Autodesk Inventor part; units mm, degrees
ref_plane "Work Plane1" through (30, 0, 0) normal (0, -0.5, 0.866) x (1, 0, 0)
ref_plane "YZ Plane" through (0, 0, 0) normal (1, 0, 0) x (0, 1, 0)
ref_plane "XZ Plane" through (0, 0, 0) normal (0, 1, 0) x (-1, 0, 0)
sketch "Sketch1" plane through (0, 0, 0) normal (0, 0, 1) x (1, 0, 0)
  line L0 (0.1133, 0) -> (20, 0)
  line L1 (20, 0) -> (20, 3)
  line L2 (20, 3) -> (2, 3)
  line L3 (2, 3) -> (1.3865, 3)
  line L4 (1.3865, 3) -> (0, 3)
  line L5 (0, 3) -> (0, 5.25)
  line L6 (0, 5.25) -> (-3.3, 5.25)
  line L7 (-3.3, 5.25) -> (-3.3, 2.3094)
  line L8 (-3.3, 2.3094) -> (-1.22, 2.3094)
  line L9 (-1.22, 2.3094) -> (0.1133, 0)
  line L10 (-7.96, 0) -> (24.66, 0)
  line L11 (0, -1.05) -> (0, 6.3)
  line L12 (2, 3) -> (0, 3) construction
  dimension "d0" = 18
  dimension "d1" = 0.6135
  dimension "d2" = 3.3
  dimension "d3" = 2.08
  dimension "d4" = 60
  dimension "d5" = 6
  dimension "d6" = 6
  dimension "d7" = 4.6188
  dimension "d8" = 10.5
  dimension "d19" = 20
revolve "Body" add sketch "Sketch1" angle 360 about axis through (0.1133, 0, 0) along (1, 0, 0) contours L9 L11 L4 L3 L2 L1 L0 | L9 L8 L7 L6 L5 L11
sketch "Sketch2" plane through (-3.3, 0, 0) normal (-1, 0, 0) x (0, 0, 1)
  circle A0 centre (0, 0) radius 2.3094
  line L0 (0, -7.35) -> (0, 7.35)
  line L1 (-7.35, 0) -> (7.35, 0)
  line L2 (2.3094, 0) -> (1.1547, -2)
  line L3 (1.1547, -2) -> (-1.1547, -2)
  line L4 (-1.1547, -2) -> (-2.3094, 0)
  line L5 (-2.3094, 0) -> (-1.1547, 2)
  line L6 (-1.1547, 2) -> (1.1547, 2)
  line L7 (1.1547, 2) -> (2.3094, 0)
extrude "Slot" add sketch "Sketch2" against normal up to next contours L7 A0 | A0 L2 | L6 L0 A0 | A0 L0 L3 | L0 L6 A0 | A0 L3 L0 | L4 A0 | A0 L5
fillet "Fillet1" radius 2.5 1 edges at (-3.3, -5.25, 0)
thread "Thread"
chamfer "Chamfer1" distance 0.6135 distance2 0.6135 1 edges at (20, -3, 0) measured on face at (20, 1.0659, 1.0214)
fillet "Fillet2" radius 0.25 1 edges at (0, -3, 0)
ref_plane "Work Plane1" through (30, 0, 0) normal (0, -0.5, 0.866) x (1, 0, 0)
equation "\"d0\" = GEL"
equation "\"d1\" = GAL"
equation "\"d2\" = KOH"
equation "\"d3\" = INTI"
equation "\"d5\" = GD"
equation "\"d6\" = BDM"
equation "\"d7\" = 1.1547 * SW"
equation "\"d8\" = KOD"
equation "\"d19\" = NLG"
equation "\"d16\" = RR"
equation "\"d12\" = GEL"
equation "\"d14\" = -0.5 * SPD + 0.5 * GD"
equation "\"d15\" = GUL"
equation "\"d29\" = R"
equation "\"GD\" = NND"
equation "\"NLG\" = 20"
equation "\"GEL\" = 18"
equation "\"KOD\" = 10.5"
equation "\"KOH\" = 3.3"
equation "\"INTI\" = 2.08"
equation "\"GAL\" = 0.61345 * PTC"
equation "\"GUL\" = 0.61345 * PTC"
equation "\"BDM\" = NND"
equation "\"SW\" = 4"
equation "\"RR\" = 2.5"
equation "\"SPD\" = 4.7731"
equation "\"d28\" = R"
equation "\"R\" = 0.25"
equation "\"TOA\" = 30deg"
equation "\"THREADDIA\" = 6"
equation "\"KOD1\" = KOD - 2 * RR"
equation "\"PTC\" = 1"
equation "\"NND\" = 6"
equation "\"E0\" = 1.155 * SW"
equation "\"GD1\" = THREADDIA - 1.2269 * PTC"
properties part number "ANSI B18.3.4M - M6 x 1 x 20, FHSBHCSM" material "Steel, Mild"
Geometry check sheet. Reference: the model listing, model coordinates, mm. A direction names the side the tool comes from. Give positions to 0.01 mm unless a question says otherwise; leave off trailing zeros. Order: outer loops, then holes, each group sorted by start corner. A loop starts at its lowest first (then second) coordinate and runs counter-clockwise, first axis right, second up. Notation, with made-up numbers: M 47,32 L 72,32 A20 cw 72,47 Z; hole C -35,-18 d9. An arc over 180 degrees is marked long. Use a Markdown table: item, result.
Item 1: Section check A-A (x = 13.5). Record the cut outline in (y, z).
Answers follow:
| item | result |
|---|---|
| outline | C 0,0 d6 |
Item 2: Depth check by flat-ended pin: P1, Ø1.5, axis at x = 5, z = 2.5, coming from the -Y side; P2, Ø0.7, axis at x = -1.5, z = 0, coming from the +Y side; P3, Ø1, axis at x = 11, y = -0.5, coming from the -Z side. Enter the tip coordinate at first touch or a pass-through.
Answers follow:
| item | result |
|---|---|
| P1 | stops at y = -2.44 |
| P2 | stops at y = 5.23 |
| P3 | stops at z = -3 |
Item 3: Material ranges on line 1 along X through (y, z) = (1.75, -2.75); line 2 along X through (y, z) = (0.25, 2); line 3 along Y through (x, z) = (3.5, 1), recorded low to high.
Answers follow:
| item | result |
|---|---|
| line 1 | x = -3.25 to 0 |
| line 2 | x = -1.05 to 20 |
| line 3 | y = -2.83 to 2.83 |
Item 4: Tool access check on faces 4 (the flat face through (-2, 2, 0)), 5 (the flat face through (20, 0, 0)). Record the directions out of +Z, -Z, +X, -X, +Y, -Y that give a thin tool (end or side, any length) a straight path to the whole face; none if there is none.
Answers follow:
| item | result |
|---|---|
| face 4 | -X |
| face 5 | +Z, -Z, +X, +Y, -Y |
Item 5: Draft check along Y on faces 1 (the flat face through (0, -0.1, -3.4)), 2 (the cylindrical face through (10, -3, 0)), 3 (the conical face through (0.03, 0.14, -0.04)). Enter one of: +Y half, -Y half, draft (parallel to the pull), parting line (faces both ways), or undercut.
Answers follow:
| item | result |
|---|---|
| face 1 | draft |
| face 2 | parting line |
| face 3 | undercut |
